```python
from build123d import *

# Parameters (mm, degrees)
EXTRUDE_1_DEPTH     = 15
EXTRUDE_1_2_DEPTH   = 15
SKETCH_1_W          = 55
SKETCH_1_H          = 4
EXTRUDE_1_3_DEPTH   = 15
SKETCH_2_W          = 55
SKETCH_2_H          = 23
SKETCH_2_W_2        = 23
SKETCH_2_H_2        = 16
EXTRUDE_2_DEPTH     = 4
SKETCH_3_R          = 2
CUT_EXTRUDE_1_DEPTH = 4


with BuildPart() as part:
    # Sketch 1 → Extrude 1 (new body)
    with BuildSketch(Plane(origin=(0, 0, 0), x_dir=(1, 0, 0), z_dir=(0, 1, 0))):
        Polygon((-13.428571429, 15.821428571), (-29.428571429, 15.821428571), (-29.428571429, 11.821428571), (-11.428571429, 11.821428571), (-9.428571429, 11.821428571), (-9.428571429, 15.821428571), (-9.428571429, 31.821428571), (-13.428571429, 31.821428571), align=None)
    extrude(amount=EXTRUDE_1_DEPTH)



with BuildPart() as body_2:
    # Sketch 1 → Extrude 1 2 (new body)
    with BuildSketch(Plane(origin=(0, 0, 0), x_dir=(1, 0, 0), z_dir=(0, 1, 0))):
        Polygon((9.571428571, 31.821428571), (5.571428571, 31.821428571), (5.571428571, 15.821428571), (5.571428571, 11.821428571), (14.214285714, 11.821428571), (25.571428571, 11.821428571), (25.571428571, 15.821428571), (9.571428571, 15.821428571), align=None)
    extrude(amount=EXTRUDE_1_2_DEPTH)


with BuildPart() as body_3:
    # Sketch 1 → Extrude 1 3 (new body)
    with BuildSketch(Plane(origin=(0, 0, 0), x_dir=(1, 0, 0), z_dir=(0, 1, 0))):
        with Locations((-1.928571429, -5.178571429)):
            Rectangle(SKETCH_1_W, SKETCH_1_H)
    extrude(amount=EXTRUDE_1_3_DEPTH)


with BuildPart() as part_1:
    add(part.part)

    add(body_2.part)  # Extrude 2 merges body 2

    add(body_3.part)  # Extrude 2 merges body 3
    # Sketch 2 → Extrude 2 (add)
    with BuildSketch(Plane(origin=(0, 15, 0), x_dir=(1, 0, 0), z_dir=(0, 1, 0))):
        with Locations((-1.928571429, 4.321428571)):
            Rectangle(SKETCH_2_W, SKETCH_2_H)
        with Locations((-1.928571429, 23.821428571)):
            Rectangle(SKETCH_2_W_2, SKETCH_2_H_2)
    extrude(amount=EXTRUDE_2_DEPTH)

    # Sketch 3 → Cut-Extrude 1 (cut)
    with BuildSketch(Plane(origin=(0, 19, 0), x_dir=(1, 0, 0), z_dir=(0, 1, 0))):
        with Locations((-1.928571429, 24.321428571)):
            Circle(SKETCH_3_R)
        with Locations((-1.928571429, 4.321428571)):
            Circle(SKETCH_3_R)
    extrude(amount=-CUT_EXTRUDE_1_DEPTH, mode=Mode.SUBTRACT)


solid = part_1.part
```
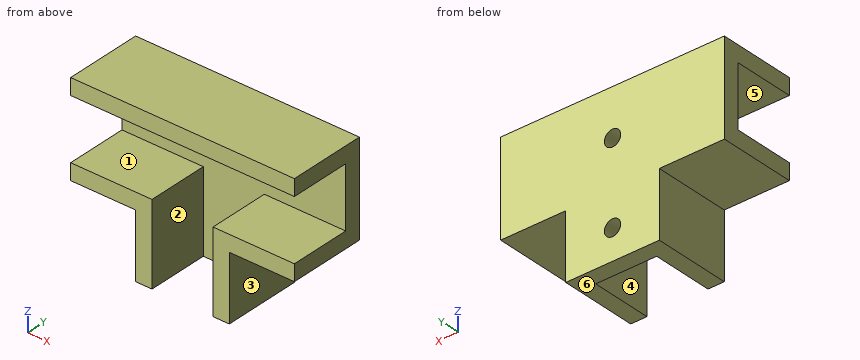
Geometry check sheet. Reference: the model listing, model coordinates, mm. Face numbers are marked on the shaded views. A direction names the side the tool comes from. Give positions to 0.01 mm unless a question says otherwise; leave off trailing zeros. Write each loop counter-clockwise with the first axis right and the second up, starting at its lowest first coordinate (ties: lowest second). Pieces come first, ordered by that corner, then holes.
1) Section check A-A, the plane y = 7.75. Record the boundary of the cut face in (x, z).
2) Section check B-B, the plane z = -20.5. Record the boundary of the cut face in (x, y), and give its area (3 significant figures).
3) Material ranges on L1, parallel to Z at x = -10.5, y = 1.25; L2, parallel to X at y = 8.5, z = -14.5; L3, parallel to X at y = 2.5, z = -28, recorded low to high.
4) Gauge pin test, flat ends, axial feed: pin 1 (4.5 mm diameter, centred on y = 10.5, z = -22.5, fed in from -X); pin 2 (5 mm diameter, centred on y = 5.5, z = -20.5, fed in from +X); pin 3 (1.5 mm diameter, centred on x = 14, y = 8.5, fed in from -Z). Record the tip position at first contact, or that the pin passes through.
5) Section check D-D, the plane z = -3. Record the boundary of the cut face in (x, y).
6) Release check for a two-part mould opening along Z. For the marked faces 4, 5 and 6 record: pulls with the +Z half, pulls with the -Z half, needs draft (parallel to the pull), parting line crosses it, or undercut.
7) Access from +Z, -Z, +X, -X, +Y, -Y to the whole of each face (thin tool, end or side, straight path). Record for the marked faces 1, 2 and 3.
8) Section check C-C, the plane x = -22. Record the boundary of the cut face in (y, z), and give its area (3 significant figures).
Computed:
1. outline: (-29.43, -15.82) - (-13.43, -15.82) - (-13.43, -31.82) - (-9.43, -31.82) - (-9.43, -11.82) - (-29.43, -11.82) - close; (-29.43, 3.18) - (25.57, 3.18) - (25.57, 7.18) - (-29.43, 7.18) - close; (5.57, -31.82) - (9.57, -31.82) - (9.57, -15.82) - (25.57, -15.82) - (25.57, -11.82) - (5.57, -11.82) - close
2. outline: (-13.43, 0) - (-9.43, 0) - (-9.43, 15) - (5.57, 15) - (5.57, 0) - (9.57, 0) - (9.57, 19) - (-13.43, 19) - close
2. area: 212 mm2
3. L1: z = -31.82 to -11.82, 3.18 to 7.18
3. L2: x = -29.43 to -9.43, 5.57 to 25.57
3. L3: x = -13.43 to -9.43, 5.57 to 9.57
4. pin 1: stops at x = -13.43
4. pin 2: stops at x = 9.57
4. pin 3: stops at z = -15.82
5. outline: (-29.43, 15) - (-3.43, 15) - (-3.43, 19) - (-29.43, 19) - close; (-0.43, 15) - (25.57, 15) - (25.57, 19) - (-0.43, 19) - close
6. face 4: needs draft
6. face 5: undercut
6. face 6: pulls with the -Z half
7. face 1: +X, -X, -Y
7. face 2: -Z, -Y
7. face 3: -Z, +X, +Y, -Y
8. outline: (0, -15.82) - (19, -15.82) - (19, 7.18) - (0, 7.18) - (0, 3.18) - (15, 3.18) - (15, -11.82) - (0, -11.82) - close
8. area: 212 mm2
